CAD build for the part. Positions are in the model's coordinates, mm. Round coordinates to 2 decimals unless told otherwise and drop trailing zeros. Loops run counter-clockwise (first coordinate to the right, second up) from the corner with the lowest first, then second, coordinate; pieces in that order, holes last. Notation, with made-up numbers: M 14,-1.5 L 36,-1.5 A23 ccw 36,13.5 Z; hole C 5,64 d1. An arc over 180 degrees is marked long. Use one line per item in the form item = value.
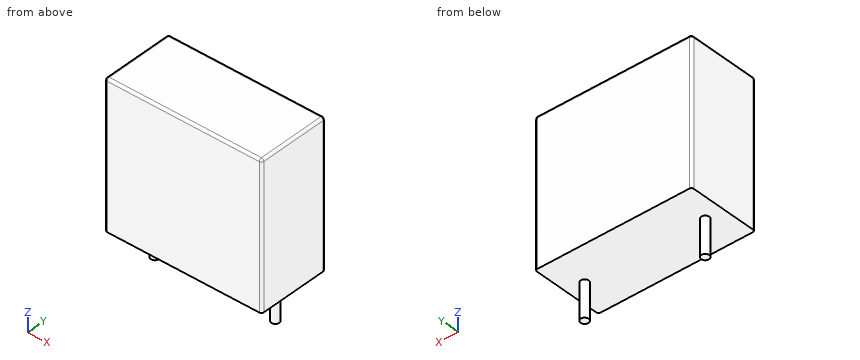
from build123d import *

# Parameters (mm, degrees)
CYLINDER001_R     = 0.33
CYLINDER001_DEPTH = 3
CYLINDER_R        = 0.33
CYLINDER_DEPTH    = 3
BOX_W             = 13
BOX_H             = 6
BOX_DEPTH         = 12
FILLET_R          = 0.2


with BuildPart() as pin2:
    # Cylinder001 → Cylinder001 (new body)
    with BuildSketch(Plane(origin=(5, 0, -3), x_dir=(1, 0, 0), z_dir=(0, 0, 1))):
        Circle(CYLINDER001_R)
    extrude(amount=CYLINDER001_DEPTH)


with BuildPart() as pin1:
    # Cylinder → Cylinder (new body)
    with BuildSketch(Plane(origin=(-5, 0, -3), x_dir=(1, 0, 0), z_dir=(0, 0, 1))):
        Circle(CYLINDER_R)
    extrude(amount=CYLINDER_DEPTH)


with BuildPart() as obj1:
    # Box → Box (new body)
    with BuildSketch(Plane(origin=(-6.5, -3, 0), x_dir=(1, 0, 0), z_dir=(0, 0, 1))):
        with Locations((6.5, 3)):
            Rectangle(BOX_W, BOX_H)
    extrude(amount=BOX_DEPTH)

    # Fillet
    fillet_edges = [obj1.edges().sort_by_distance(p)[0] for p in [
        (-6.5, -3, 6),
        (-6.5, 0, 12),
        (-6.5, 3, 6),
        (6.5, -3, 6),
        (6.5, 0, 12),
        (6.5, 3, 6),
        (0, -3, 12),
        (0, 3, 12),
    ]]
    fillet(fillet_edges, radius=FILLET_R)

    # Fusion: union Pin1
    add(pin1.part)

    # Fusion001: union Pin2
    add(pin2.part)


solid = obj1.part
1. Cut at B-B on y = 0. Write the cut outline in (x, z), and give its area (3 significant figures).
Completed:
outline = M -6.5,0 L -5.33,0 L -5.33,-3 L -4.67,-3 L -4.67,0 L 4.67,0 L 4.67,-3 L 5.33,-3 L 5.33,0 L 6.5,0 L 6.5,11.8 A0.2 ccw 6.3,12 L -6.3,12 A0.2 ccw -6.5,11.8 Z
area = 160 mm2
2. Cut at C-C on x = -1.5. Write the cut outline in (y, z), and give its area (3 significant figures).
Completed:
outline = M -3,0 L 3,0 L 3,11.8 A0.2 ccw 2.8,12 L -2.8,12 A0.2 ccw -3,11.8 Z
area = 72.0 mm2
3. Cut at D-D on y = -1.65. Write the cut outline in (x, z), and give its area (3 significant figures).
Completed:
outline = M -6.5,0 L 6.5,0 L 6.5,11.8 A0.2 ccw 6.3,12 L -6.3,12 A0.2 ccw -6.5,11.8 Z
area = 156 mm2
4. Drop a flat-ended pin along its axis: P1, Ø1.5, axis at x = -1.5, y = 2.5, coming from the -Z side. Give the stop position or say it passes through.
Completed:
P1 = 0
5. Cut at A-A on x = -5. Write the cut outline in (y, z), and give its area (3 significant figures).
Completed:
outline = M -3,0 L -0.33,0 L -0.33,-3 L 0.33,-3 L 0.33,0 L 3,0 L 3,11.8 A0.2 ccw 2.8,12 L -2.8,12 A0.2 ccw -3,11.8 Z
area = 74.0 mm2
6. Probe line 1 along Z through (x, y) = (1.25, -0.6). List the from-to ranges inside material, lowest first. Write a range as from..to.
Completed:
line_1 = 0..12
